Part model, mm, in its own coordinate system. Give positions to 0.01 mm unless a question says otherwise; leave off trailing zeros. Write each loop counter-clockwise with the first axis right and the second up, starting at its lowest first coordinate (ties: lowest second). Pieces come first, ordered by that corner, then holes.
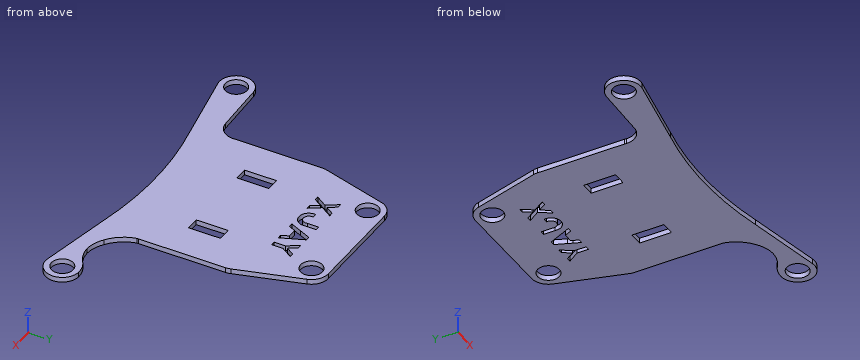
```python
from build123d import *

# Parameters (mm, degrees)
F0_R     = 6.5
F1_DEPTH = 3


with BuildPart() as f1:
    # F0 (on Top) → F1 (new body)
    with BuildSketch(Plane.XY):
        with BuildLine():
            ThreePointArc((-50.4446934155, 54.643037695), (-50.7311517832, 53.2865797574), (-50.8272536099, 51.9035392764))
            Line((-50.8272536099, 51.9035392764), (-50.8272536099, 0))
            Line((-50.8272536099, 0), (-50.793080697, -0.9064006647))
            ThreePointArc((-50.793080697, -0.9064006647), (-53.4535309431, -8.0827958775), (-60.4092310726, -11.2760511869))
            Line((-60.4092310726, -11.2760511869), (-91.7179190296, -12.4564442613))
            ThreePointArc((-91.7179190296, -12.4564442613), (-101.3019147634, -23.5749788423), (-89.4783611915, -32.2743102182))
            Line((-89.4783611915, -32.2743102182), (-44.7528083417, -23.6906495904))
            ThreePointArc((-44.7528083417, -23.6906495904), (-0.027288473, -18.9100440737), (44.6982313957, -23.6906495904))
            Line((44.6982313957, -23.6906495904), (89.4018683635, -32.2701168083))
            ThreePointArc((89.4018683635, -32.2701168083), (101.2221357059, -23.5834967295), (91.6636327073, -12.4564526987))
            ThreePointArc((91.6636327073, -12.4564526987), (86.6833273054, -13.1568395353), (82.2565257549, -15.5437646806))
            ThreePointArc((82.2565257549, -15.5437646806), (77.0307926492, -18.0592618118), (71.3056156264, -18.9857392083))
            ThreePointArc((71.3056156264, -18.9857392083), (65.5296199383, -17.9121006865), (60.3547054978, -15.1308983568))
            ThreePointArc((60.3547054978, -15.1308983568), (54.175499635, -8.9454500235), (50.73856136, -0.9061831743))
            Line((50.73856136, -0.9061831743), (50.7727463901, 0))
            Line((50.7727463901, 0), (50.7727463901, 51.8538707076))
            ThreePointArc((50.7727463901, 51.8538707076), (50.669793885, 53.2851117367), (50.3630562134, 54.6868827959))
            Line((50.3630562134, 54.6868827959), (38.8602722461, 93.6260961278))
            ThreePointArc((38.8602722461, 93.6260961278), (35.256191583, 98.8033936741), (29.2699624228, 100.7930840395))
            Line((29.2699624228, 100.7930840395), (-29.7496853037, 100.7930840395))
            ThreePointArc((-29.7496853037, 100.7930840395), (-35.7748415596, 98.7741549008), (-39.3671251094, 93.5325824581))
            Line((-39.3671251094, 93.5325824581), (-50.4446934155, 54.643037695))
        make_face()
        with Locations((-91.3411689563, -22.4493447103)):
            Circle(F0_R, mode=Mode.SUBTRACT)
        Polygon((-21.4136268049, 36.65), (-21.4136268049, 26.65), (-21.4136268049, 17.65), (-29.4136268049, 17.65), (-29.4136268049, 26.65), (-29.4136268049, 36.65), align=None, mode=Mode.SUBTRACT)
        with Locations((91.2866589082, -22.4493447103)):
            Circle(F0_R, mode=Mode.SUBTRACT)
        Polygon((21.3863731951, 17.65), (21.3863731951, 26.65), (21.3863731951, 36.65), (29.3863731951, 36.65), (29.3863731951, 26.65), (29.3863731951, 17.65), align=None, mode=Mode.SUBTRACT)
        Polygon((-22.8592688218, 69.2477548305), (-27.2865649313, 76.0405882364), (-24.7233938426, 76.0405882364), (-21.5776832774, 71.2141010795), (-18.4319727123, 76.0405882364), (-15.8688016236, 76.0405882364), (-20.2960977331, 69.2477548305), (-15.8688016236, 62.4549214246), (-18.4319727123, 62.4549214246), (-21.5776832774, 67.2814085815), (-24.7233938426, 62.4549214246), (-27.2865649313, 62.4549214246), align=None, mode=Mode.SUBTRACT)
        with BuildLine():
            ThreePointArc((-1.7979582322, 69.2477548305), (-7.5129582322, 62.4999219931), (-13.2279582322, 69.2477548305))
            Line((-13.2279582322, 69.2477548305), (-10.6625582322, 69.2477548305))
            ThreePointArc((-10.6625582322, 69.2477548305), (-7.5129582322, 65.1356067586), (-4.3633582322, 69.2477548305))
            Line((-4.3633582322, 69.2477548305), (-4.3633582322, 76.0405882364))
            Line((-4.3633582322, 76.0405882364), (-1.7979582322, 76.0405882364))
            Line((-1.7979582322, 76.0405882364), (-1.7979582322, 69.2477548305))
        make_face(mode=Mode.SUBTRACT)
        with Locations((-29.7496853037, 90.7930840395)):
            Circle(F0_R, mode=Mode.SUBTRACT)
        Polygon((2.5654, 62.4549214246), (0, 62.4549214246), (3.0334836338, 69.2477548305), (6.0669672675, 76.0405882364), (8.6323672675, 76.0405882364), (11.4274396446, 69.2477548305), (12.4830343056, 66.6823548305), (14.2225120217, 62.4549214246), (11.6571120217, 62.4549214246), (9.9176343056, 66.6823548305), (4.453249927, 66.6823548305), align=None, mode=Mode.SUBTRACT)
        Polygon((18.6675120217, 69.2282911245), (14.2225120217, 76.0405882364), (16.7879120217, 76.0405882364), (19.9375120217, 71.21358914), (23.0871120217, 76.0405882364), (25.6525120217, 76.0405882364), (21.2075120217, 69.2282911245), (21.2075120217, 62.4549214246), (19.9375120217, 62.4549214246), (18.6675120217, 62.4549214246), align=None, mode=Mode.SUBTRACT)
        with Locations((29.2699624228, 90.7930840395)):
            Circle(F0_R, mode=Mode.SUBTRACT)
    extrude(amount=F1_DEPTH)


solid = f1.part
```
1) Saw through at D-D, the plane x = 75.5. Write the cut outline in (y, z).
Answers follow:
outline: (-29.6, 0) - (-18.48, 0) - (-18.48, 3) - (-29.6, 3) - close
2) Pin check, flat tips, straight feed: pin 1 Ø1.5 at (y, z) = (57.5, 2) entering from -X; pin 2 Ø0.8 at (x, z) = (7.5, 2) entering from -Y; pin 3 Ø0.8 at (x, z) = (-26, 2) entering from -Y. Stop position of each tip, or through.
Answers follow:
pin 1: stops at x = -49.84
pin 2: stops at y = -19.06
pin 3: stops at y = -20.56
3) Saw through at A-A, the plane y = 21. Write the cut outline in (x, z), then the cut area to 3 significant figures.
Answers follow:
outline: (-50.83, 0) - (-29.41, 0) - (-29.41, 3) - (-50.83, 3) - close; (-21.41, 0) - (21.39, 0) - (21.39, 3) - (-21.41, 3) - close; (29.39, 0) - (50.77, 0) - (50.77, 3) - (29.39, 3) - close
area: 257 mm2
4) Wall check: L1, parallel to X at y = 35.5, z = 1.45; L2, parallel to X at y = 87.5, z = 2.7; L3, parallel to Y at x = -27, z = 0.9. Give the ranges that are in metal, low to high.
Answers follow:
L1: x = -50.83 to -29.41, -21.41 to 21.39, 29.39 to 50.77
L2: x = -41.09 to -35.35, -24.15 to 23.67, 34.87 to 40.67
L3: y = -20.64 to 17.65, 36.65 to 62.45, 62.89 to 75.6, 76.04 to 84.9, 96.68 to 100.79
5) Saw through at C-C, the plane y = 48. Write the cut outline in (x, z).
Answers follow:
outline: (-50.83, 0) - (50.77, 0) - (50.77, 3) - (-50.83, 3) - close
6) Saw through at B-B, the plane z = 0.95. Count the separate pieces of the cut face and the enclosed holes in it, then the cut area to 3 significant figures.
Answers follow:
separate pieces: 1
enclosed holes: 10
area: 12,200 mm2
